```python
from build123d import *

# Parameters (mm, degrees)
SKETCH_1_W          = 8
SKETCH_1_H          = 8
EXTRUDE_1_DEPTH     = 9.6
SKETCH_2_W          = 1.6
SKETCH_2_H          = 8
CUT_EXTRUDE_1_DEPTH = 8
SKETCH_5_R          = 2.4
EXTRUDE_2_DEPTH     = 1.8
SKETCH_8_R          = 1.6
CUT_EXTRUDE_3_DEPTH = 9
SKETCH_9_R          = 2.4
EXTRUDE_3_DEPTH     = 1.8
SKETCH_13_W         = 4.8
SKETCH_13_H         = 4.803439306
CUT_EXTRUDE_4_DEPTH = 5
SKETCH_15_R         = 2.5
CUT_EXTRUDE_5_DEPTH = 1.8


with BuildPart() as part:
    # Эскиз1 → Бобышка-Вытянуть1 (new body)
    with BuildSketch(Plane(origin=(0, 0, 0), x_dir=(1, 0, 0), z_dir=(0, 1, 0))):
        Rectangle(SKETCH_1_W, SKETCH_1_H)
    extrude(amount=EXTRUDE_1_DEPTH)

    # Эскиз2 → Вырез-Вытянуть1 (cut)
    with BuildSketch(Plane(origin=(0, 9.6, 0), x_dir=(1, 0, 0), z_dir=(0, 1, 0))):
        with Locations((3.2, 0)):
            Rectangle(SKETCH_2_W, SKETCH_2_H)
    extrude(amount=-CUT_EXTRUDE_1_DEPTH, mode=Mode.SUBTRACT)

    # Эскиз5 → Бобышка-Вытянуть2 (add)
    with BuildSketch(Plane(origin=(2.4, 0, 0), x_dir=(0, 0, -1), z_dir=(1, 0, 0))):
        with Locations(Location((0, 5.6, 0), (0, 0, 180))):
            Circle(SKETCH_5_R)
    extrude(amount=EXTRUDE_2_DEPTH)

    # Эскиз8 → Вырез-Вытянуть3 (cut)
    with BuildSketch(Plane(origin=(4.2, 0, 0), x_dir=(0, 0, -1), z_dir=(1, 0, 0))):
        with Locations((0, 5.6)):
            Circle(SKETCH_8_R)
    extrude(amount=-CUT_EXTRUDE_3_DEPTH, mode=Mode.SUBTRACT)

    # Эскиз9 → Бобышка-Вытянуть3 (add)
    with BuildSketch(Plane(origin=(0, 9.6, 0), x_dir=(1, 0, 0), z_dir=(0, 1, 0))):
        Circle(SKETCH_9_R)
    extrude(amount=EXTRUDE_3_DEPTH)

    # Эскиз13 → Вырез-Вытянуть4 (cut)
    with BuildSketch(Plane.ZY.offset(4)):
        with Locations((0, 5.6)):
            Rectangle(SKETCH_13_W, SKETCH_13_H)
    extrude(amount=-CUT_EXTRUDE_4_DEPTH, mode=Mode.SUBTRACT)

    # Эскиз15 → Вырез-Вытянуть5 (cut)
    with BuildSketch(Plane.XZ):
        with Locations(Location((0, 0, 0), (0, 0, 270))):
            Circle(SKETCH_15_R)
    extrude(amount=-CUT_EXTRUDE_5_DEPTH, mode=Mode.SUBTRACT)


solid = part.part
```
CAD build for the part. Positions are in the model's coordinates, mm. A direction names the side the tool comes from. Round coordinates to 2 decimals unless told otherwise and drop trailing zeros. Write each loop counter-clockwise with the first axis right and the second up, starting at its lowest first coordinate (ties: lowest second). Pieces come first, ordered by that corner, then holes.
Item 1: Band-saw the part on C-C on z = 1. Write the cut outline in (x, y).
Filled in:
outline: (-4, 0) - (-2.29, 0) - (-2.29, 1.8) - (2.29, 1.8) - (2.29, 0) - (4, 0) - (4, 1.6) - (2.4, 1.6) - (2.4, 3.42) - (4.2, 3.42) - (4.2, 4.35) - (1, 4.35) - (1, 3.2) - (-4, 3.2) - close; (-4, 8) - (1, 8) - (1, 6.85) - (4.2, 6.85) - (4.2, 7.78) - (2.4, 7.78) - (2.4, 9.6) - (2.18, 9.6) - (2.18, 11.4) - (-2.18, 11.4) - (-2.18, 9.6) - (-4, 9.6) - close
Item 2: Drop flat-ended pins along their axis: pin 1 Ø3 at (x, z) = (1, -2.5) entering from -Y; pin 2 Ø1.3 at (x, z) = (3.5, 1.5) entering from +Y; pin 3 Ø0.5 at (y, z) = (0.5, 0) entering from +X; pin 4 Ø1.4 at (x, z) = (-1.5, 0.5) entering from -Y. Give the stop position or say it passes through.
Filled in:
pin 1: stops at y = 0
pin 2: stops at y = 7.84
pin 3: stops at x = 4
pin 4: stops at y = 1.8
Item 3: Tool access for faces 1 (the flat face through (1, 6, -2)), 2 (the cylindrical face through (-2.44, 0.89, 0.54)), 3 (the cylindrical face through (3.287, 7.943, -0.52)): list every direction of +Z, -Z, +X, -X, +Y, -Y with a clear straight run to the whole face (end or side of a thin tool).
Filled in:
face 1: -X
face 2: -Y
face 3: +X
Item 4: Band-saw the part on B-B on x = 3.5. Write the cut outline in (y, z).
Filled in:
outline: (0, -4) - (1.6, -4) - (1.6, 4) - (0, 4) - close; circle Ø4.8 at (5.6, 0); hole circle Ø3.2 at (5.6, 0)
Item 5: Band-saw the part on D-D on x = 0. Write the cut outline in (y, z).
Filled in:
outline: (0, -4) - (9.6, -4) - (9.6, -2.4) - (11.4, -2.4) - (11.4, 2.4) - (9.6, 2.4) - (9.6, 4) - (0, 4) - (0, 2.5) - (1.8, 2.5) - (1.8, -2.5) - (0, -2.5) - close; hole (3.2, -2.4) - (8, -2.4) - (8, 2.4) - (3.2, 2.4) - close
Item 6: Drill centre lines: L1, parallel to Y at x = 2.75, z = 0; L2, parallel to X at y = 0.55, z = 0; L3, parallel to Y at x = -0.5, z = -2.25. Where is each one in solid material? Low to high.
Filled in:
L1: y = 0 to 1.6, 3.2 to 4, 7.2 to 8
L2: x = -4 to -2.5, 2.5 to 4
L3: y = 1.8 to 3.2, 8 to 11.4
Item 7: Mould opens along Z. For faces 4 (the flat face through (2.4, 4, 2)), 5 (the flat face through (-2, 3.198, 0)), 6 (the flat face through (-2, 6, 2.4)), 7 (the cylindrical face through (1.29, 10.487, -2.024)) say: released by +Z, released by -Z, zero draft, split by the parting line, or undercut.
Filled in:
face 4: zero draft
face 5: undercut
face 6: undercut
face 7: split by the parting line
Item 8: Band-saw the part on A-A on y = 5.6. Write the cut outline in (x, z), then the cut area to 3 significant figures.
Filled in:
outline: (-4, -4) - (2.4, -4) - (2.4, -2.4) - (4.2, -2.4) - (4.2, -1.6) - (1, -1.6) - (1, -2.4) - (-4, -2.4) - close; (-4, 2.4) - (1, 2.4) - (1, 1.6) - (4.2, 1.6) - (4.2, 2.4) - (2.4, 2.4) - (2.4, 4) - (-4, 4) - close
area: 25.6 mm2
